from build123d import *

# Parameters (mm, degrees)
F1_DEPTH  = 10
F2_R      = 4
F3_W      = 10
F3_H      = 26
F4_DEPTH  = 31
F5_R      = 6.5
F6_DEPTH  = 69.001
F7_R      = 6.5
F8_DEPTH  = 69.001
F9_W      = 20
F9_H      = 12
F10_DEPTH = 26


with BuildPart() as f1:
    # F0 (on Top) → F1 (new body)
    with BuildSketch(Plane.XY):
        with BuildLine():
            Line((-9, 140), (-25, 140))
            ThreePointArc((-25, 140), (-43.384776, 132.384776), (-51, 114))
            Line((-51, 114), (-51, -114))
            ThreePointArc((-51, -114), (-43.384776, -132.384776), (-25, -140))
            Line((-25, -140), (-9, -140))
            Line((-9, -140), (-9, -125))
            ThreePointArc((-9, -125), (-6.363961, -118.636039), (0, -116))
            ThreePointArc((0, -116), (6.363961, -118.636039), (9, -125))
            Line((9, -125), (9, -140))
            Line((9, -140), (25, -140))
            ThreePointArc((25, -140), (43.384776, -132.384776), (51, -114))
            Line((51, -114), (51, 114))
            ThreePointArc((51, 114), (43.384776, 132.384776), (25, 140))
            Line((25, 140), (9, 140))
            Line((9, 140), (9, 125))
            ThreePointArc((9, 125), (6.363961, 118.636039), (0, 116))
            ThreePointArc((0, 116), (-6.363961, 118.636039), (-9, 125))
            Line((-9, 125), (-9, 140))
        make_face()
    extrude(amount=F1_DEPTH)

    # F2
    f2_edges = [f1.edges().sort_by_distance(p)[0] for p in [
        (-9, -140, 5),
        (9, -140, 5),
        (-9, 140, 5),
        (9, 140, 5),
    ]]
    fillet(f2_edges, radius=F2_R)

    # F3 (on face) → F4 (join)
    with BuildSketch(Plane.XY.offset(10)):
        with Locations((13, -91)):
            Rectangle(F3_W, F3_H)
        with Locations((-13, -91)):
            Rectangle(F3_W, F3_H)
        with Locations((-13, 91)):
            Rectangle(F3_W, F3_H)
        with Locations((13, 91)):
            Rectangle(F3_W, F3_H)
    extrude(amount=F4_DEPTH)

    # F5 (on face) → F6 (cut, through all)
    with BuildSketch(Plane.YZ.offset(18)):
        with Locations((-91, 28)):
            Circle(F5_R)
        with BuildLine():
            Line((-78, 41), (-91, 41))
            ThreePointArc((-91, 41), (-81.807612, 37.192388), (-78, 28))
            Line((-78, 28), (-78, 41))
        make_face()
        with BuildLine():
            Line((-104, 41), (-104, 28))
            ThreePointArc((-104, 28), (-100.192388, 37.192388), (-91, 41))
            Line((-91, 41), (-104, 41))
        make_face()
    extrude(amount=-F6_DEPTH, mode=Mode.SUBTRACT)

    # F7 (on face) → F8 (cut, through all)
    with BuildSketch(Plane.YZ.offset(18)):
        with Locations((91, 28)):
            Circle(F7_R)
        with BuildLine():
            Line((78, 41), (78, 28))
            ThreePointArc((78, 28), (81.807612, 37.192388), (91, 41))
            Line((91, 41), (78, 41))
        make_face()
        with BuildLine():
            Line((104, 41), (91, 41))
            ThreePointArc((91, 41), (100.192388, 37.192388), (104, 28))
            Line((104, 28), (104, 41))
        make_face()
    extrude(amount=-F8_DEPTH, mode=Mode.SUBTRACT)

    # F9 (on face) → F10 (join)
    with BuildSketch(Plane.XY.offset(10)):
        with Locations((41, 78)):
            Rectangle(F9_W, F9_H)
        with Locations((-41, 78)):
            Rectangle(F9_W, F9_H)
    extrude(amount=F10_DEPTH)


solid = f1.part
The listing builds one solid part. Answer for the finished solid, in the listing's coordinates (mm). A direction names the side the tool comes from. Give positions to 0.01 mm unless a question says otherwise; leave off trailing zeros. Write each loop counter-clockwise with the first axis right and the second up, starting at its lowest first coordinate (ties: lowest second). Pieces come first, ordered by that corner, then holes. Notation, with made-up numbers: (36, 15) - (60, 15) arc R15 ccw to (60, 30) - close; hole circle Ø9 at (31.25, 83.5). An arc over 180 degrees is marked (long way). Use a Markdown table: item, result.
1. Each of these flat-tipped pins is pushed along its axis until it touches: P1, Ø1, axis at x = 26.5, y = -97, coming from the +Z side; P2, Ø11, axis at y = 129, z = 4.5, coming from the +X side; P3, Ø1, axis at x = -1.5, z = 9.5, coming from the -Y side; P4, Ø8, axis at y = 91, z = 28, coming from the +X side. Where does it stop, or does it pass through?
Values follow:
| item | result |
|---|---|
| P1 | stops at z = 10 |
| P2 | stops at x = 49.2 |
| P3 | stops at y = -116.23 |
| P4 | passes through |
2. For a pull along Y with two mould halves and no side action, classify faces 1 (the flat face through (41, 84, 23)), 2 (the flat face through (-41, 72, 23)), 3 (the cylindrical face through (-12.93, -84.8, 29.95)), 4 (the flat face through (51, 23.7, 9.7)) as released by +Y, released by -Y, zero draft, split by the parting line, or undercut.
Values follow:
| item | result |
|---|---|
| face 1 | released by +Y |
| face 2 | released by -Y |
| face 3 | undercut |
| face 4 | zero draft |
3. A tool of negligible diameter and unlimited length cuts with its end or side. For faces 5 (the flat face through (9, -130, 5)), 6 (the flat face through (41, 78, 36)), 7 (the flat face through (-18, -94, 22)), 8 (the flat face through (31, 78, 23)), 9 (the flat face through (13, 104, 19)), from which of +Z, -Z, +X, -X, +Y, -Y can it reach the whole face along a straight path? Write none if from no direction.
Values follow:
| item | result |
|---|---|
| face 5 | +Z, -Z, -Y |
| face 6 | +Z, +X, +Y, -Y |
| face 7 | +Z, -X, +Y, -Y |
| face 8 | +Z, +Y, -Y |
| face 9 | +Z, +X, -X, +Y |
4. Section A-A on z = 16.5 is taken. Write down the section's boundary in (x, y), plus the area to 3 significant figures.
Values follow:
| item | result |
|---|---|
| outline | (-51, 72) - (-31, 72) - (-31, 84) - (-51, 84) - close; (-18, -104) - (-8, -104) - (-8, -78) - (-18, -78) - close; (-18, 78) - (-8, 78) - (-8, 104) - (-18, 104) - close; (8, -104) - (18, -104) - (18, -78) - (8, -78) - close; (8, 78) - (18, 78) - (18, 104) - (8, 104) - close; (31, 72) - (51, 72) - (51, 84) - (31, 84) - close |
| area | 1,520 mm² |
5. Section B-B on y = 3 is taken. Write down the section's boundary in (x, z).
Values follow:
| item | result |
|---|---|
| outline | (-51, 0) - (51, 0) - (51, 10) - (-51, 10) - close |
6. Section C-C on z = 31 is taken. Count the separate pieces of the cut face and the enclosed holes in it, plus the area to 3 significant figures.
Values follow:
| item | result |
|---|---|
| separate pieces | 10 |
| enclosed holes | 0 |
| area | 1,030 mm² |
7. Find the intervals of material crossed by probe 1 along Z at (x, y) = (13, -91); probe 2 along Z at (x, y) = (-9.5, -58.5); probe 3 along X at (y, z) = (-124.5, 2), in increasing order. Write a range as from..to.
Values follow:
| item | result |
|---|---|
| probe 1 | z = 0..21.5, 34.5..41 |
| probe 2 | z = 0..10 |
| probe 3 | x = -48.79..-8.99, 8.99..48.79 |
